Can you work these out from the model? Positions are in its coordinate system, mm. Face numbers are marked on the shaded views. A direction names the side the tool comes from. Round coordinates to 2 decimals unless told otherwise and drop trailing zeros. Order: outer loops, then holes, each group sorted by start corner. A loop starts at its lowest first (then second) coordinate and runs counter-clockwise, first axis right, second up.
Q1. We'd pull the mould along Y, two halves only. Please class the marked faces 1, 2 and 3: pulls with the +Y half, pulls with the -Y half, needs draft (parallel to the pull), parting line crosses it, or undercut.
Q2. If we section it at A-A (x = 52): Please give me the cut outline in (y, z) (3 decimals).
Q3. If I drill on line 1 (Y direction, x = 64, z = -20) (3 decimals); line 2 (Z direction, x = 194.5, y = 30) (3 decimals); line 3 (Z direction, x = 215.9, y = 35.75), over which ranges is the centre line in solid material (lowest first)?
Q4. Will these pins go through, and if not, where does the flat tip stop? P1, Ø11, axis at x = 28.58, z = -16.67, coming from the -Y side (3 decimals); P2, Ø1, axis at x = 73, y = 20, coming from the -Z side; P3, Ø22, axis at x = 193, y = 12, coming from the -Z side.
Q5. If we section it at B-B (y = 11): Please give me the cut outline in (x, z) (3 decimals), plus the area to 3 significant figures.
Q6. For the marked faces 4 and 5, which set-ups out of +Z, -Z, +X, -X, +Y, -Y let a thin tool reach every point of the face, with its end or its side?
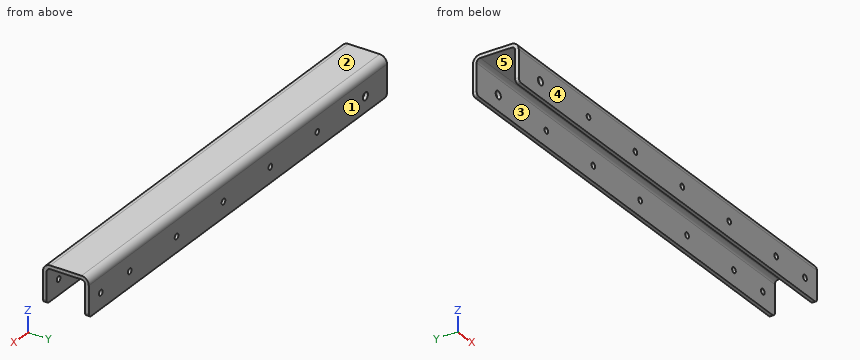
from build123d import *

# Parameters (mm, degrees)
BASE_FLANGE1_DEPTH = 393.7
SKETCH6_R          = 3.3782
SKETCH6_R_2        = 2.4257
CUT_EXTRUDE1_DEPTH = 397.892779602
FILLET1_R          = 3.175


# Sheet-metal steps are written as plain solids
with BuildPart() as part:
    # Sketch1 → Base-Flange1 (new body)
    with BuildSketch(Plane(origin=(0, 0, 0), x_dir=(0, 0, -1), z_dir=(1, 0, 0))):
        with BuildLine():
            Line((30.226, 33.782), (3.175, 33.782))
            ThreePointArc((3.175, 33.782), (0.92993597, 32.85206403), (0, 30.607))
            Line((0, 30.607), (0, 3.175))
            ThreePointArc((0, 3.175), (0.92993597, 0.92993597), (3.175, 0))
            Line((3.175, 0), (30.226, 0))
            Line((30.226, 0), (30.226, -3.175))
            Line((30.226, -3.175), (3.175, -3.175))
            ThreePointArc((3.175, -3.175), (-1.315128061, -1.315128061), (-3.175, 3.175))
            Line((-3.175, 3.175), (-3.175, 30.607))
            ThreePointArc((-3.175, 30.607), (-1.315128061, 35.097128061), (3.175, 36.957))
            Line((3.175, 36.957), (30.226, 36.957))
            Line((30.226, 36.957), (30.226, 33.782))
        make_face()
    extrude(amount=BASE_FLANGE1_DEPTH)

    # Sketch6 → Cut-Extrude1 (cut, through all)
    with BuildSketch(Plane(origin=(0, 36.957, 0), x_dir=(1, 0, 0), z_dir=(0, 1, 0))):
        with Locations(Location((28.575, 16.66875, 0), (0, 0, 270))):
            Circle(SKETCH6_R)
        with Locations(Location((92.075, 16.66875, 0), (0, 0, 270))):
            Circle(SKETCH6_R_2)
        with Locations(Location((339.725, 16.66875, 0), (0, 0, 270))):
            Circle(SKETCH6_R_2)
        with Locations(Location((377.825, 16.66875, 0), (0, 0, 270))):
            Circle(SKETCH6_R_2)
        with Locations(Location((153.9875, 16.66875, 0), (0, 0, 270))):
            Circle(SKETCH6_R_2)
        with Locations(Location((215.9, 16.66875, 0), (0, 0, 270))):
            Circle(SKETCH6_R_2)
        with Locations(Location((277.8125, 16.66875, 0), (0, 0, 270))):
            Circle(SKETCH6_R_2)
    extrude(amount=-CUT_EXTRUDE1_DEPTH, mode=Mode.SUBTRACT)

    # Fillet1
    fillet1_edges = [part.edges().sort_by_distance(p)[0] for p in [
        (0, -1.5875, -30.226),
        (0, 35.3695, -30.226),
        (393.7, -1.5875, -30.226),
        (393.7, 35.3695, -30.226),
    ]]
    fillet(fillet1_edges, radius=FILLET1_R)


solid = part.part
Solution:
1. face 1: pulls with the +Y half
1. face 2: needs draft
1. face 3: undercut
2. outline: (-3.175, -30.226) - (0, -30.226) - (0, -3.175) arc R3.175 cw to (3.175, 0) - (30.607, 0) arc R3.175 cw to (33.782, -3.175) - (33.782, -30.226) - (36.957, -30.226) - (36.957, -3.175) arc R6.35 ccw to (30.607, 3.175) - (3.175, 3.175) arc R6.35 ccw to (-3.175, -3.175) - close
3. line 1: y = -3.175 to 0, 33.782 to 36.957
3. line 2: z = 0 to 3.175
3. line 3: z = -30.23 to -19.09, -14.24 to 0.55
4. P1: stops at y = -3.175
4. P2: stops at z = 0
4. P3: stops at z = -0.86
5. outline: (0, 0) - (393.7, 0) - (393.7, 3.175) - (0, 3.175) - close
5. area: 1,250 mm2
6. face 4: +Z, -Z, +X, -X, -Y
6. face 5: -Z, +X, -X
